Autodesk Inventor part; units mm, degrees
ref_plane "YZ Plane" through (0, 0, 0) normal (1, 0, 0) x (0, 1, 0)
ref_plane "XZ Plane" through (0, 0, 0) normal (0, 1, 0) x (-1, 0, 0)
ref_plane "XY Plane" through (0, 0, 0) normal (0, 0, 1) x (1, 0, 0)
sketch "Sketch1" plane through (0, 0, 0) normal (0, 1, 0) x (-1, 0, 0)
  circle A0 centre (0, 0) radius 3
  circle A1 centre (0, 0) radius 1.5
  circle A2 centre (0, 0) radius 1.75
  circle A3 centre (0, 0) radius 2.75
  dimension "d0" = 6
  dimension "d1" = 3
  dimension "d2" = 3.5
  dimension "d3" = 5.5
extrude "Extrusion1" add sketch "Sketch1" along normal blind 2.5 contours A0 | A2 | A3
extrude "Extrusion2" cut sketch "Sketch1" against normal blind 0.1 from surface at 2.5 contours A3
extrude "Extrusion3" cut sketch "Sketch1" along normal blind 0.1 contours A3
properties part number "Miniatur Kugellager MR 63 2RS 3x6x2.5 mm"
Verification items for the finished model (mm, model axes). A direction names the side the tool comes from. Give positions to 0.01 mm unless a question says otherwise; leave off trailing zeros. Order: outer loops, then holes, each group sorted by start corner. A loop starts at its lowest first (then second) coordinate and runs counter-clockwise, first axis right, second up. Notation, with made-up numbers: M 69.5,0 L 96.5,0 A5 cw 96.5,5 Z; hole C 57.25,82.5 d4. An arc over 180 degrees is marked long. Use one line per item in the form item = value. Start each with the question number.
Q1. Section check D-D (x = -1.95). Enter the section's corners in (y, z).
Q2. Go/stop test with a flat-tipped pin: pin 1 Ø1 at (y, z) = (0.5, 2) entering from +X. Record where the tip stops, or that it passes through.
Q3. Section check C-C (y = 1). Enter the section's corners in (x, z), then the cut area to 3 significant figures.
Q4. Section check B-B (x = 0). Enter the section's corners in (y, z), then the cut area to 3 significant figures.
Q5. Mould release check, pull along Z, two halves, no side actions. Record for faces 1 (the cylindrical face through (3, 1, 0)), 2 (the flat face through (-2, 0.1, 0)): +Z half, -Z half, draft (parallel to the pull), parting line (faces both ways), or undercut.
Q6. Access from +Z, -Z, +X, -X, +Y, -Y to the whole of each face (thin tool, end or side, straight path). Record for faces 3 (the flat face through (-2, 2.4, 0)), 4 (the cylindrical face through (1.5, 1.23, -0.07)).
Q7. Scan lines: line 1 along Z through (x, y) = (0, 0.05); line 2 along Z through (x, y) = (0, 0.15). Record each from-to range of solid material in increasing order. Write a range as [from, to].
Q8. Section check A-A (z = 0). Enter the section's corners in (x, y).
Evaluation:
q1.outline = M 0,-2.28 L 2.5,-2.28 L 2.5,-1.94 L 2.4,-1.94 L 2.4,1.94 L 2.5,1.94 L 2.5,2.28 L 0,2.28 L 0,1.94 L 0.1,1.94 L 0.1,-1.94 L 0,-1.94 Z
q2.pin_1 = 2.6
q3.outline = C 0,0 d6; hole C 0,0 d3
q3.area = 21.2 mm2
q4.outline = M 0,-3 L 2.5,-3 L 2.5,-2.75 L 2.4,-2.75 L 2.4,-1.75 L 2.5,-1.75 L 2.5,-1.5 L 0,-1.5 L 0,-1.75 L 0.1,-1.75 L 0.1,-2.75 L 0,-2.75 Z; M 0,1.5 L 2.5,1.5 L 2.5,1.75 L 2.4,1.75 L 2.4,2.75 L 2.5,2.75 L 2.5,3 L 0,3 L 0,2.75 L 0.1,2.75 L 0.1,1.75 L 0,1.75 Z
q4.area = 7.10 mm2
q5.face_1 = parting line
q5.face_2 = undercut
q6.face_3 = +Y
q6.face_4 = +Y, -Y
q7.line_1 = [-3, -2.75], [-1.75, -1.5], [1.5, 1.75], [2.75, 3]
q7.line_2 = [-3, -1.5], [1.5, 3]
q8.outline = M -3,0 L -2.75,0 L -2.75,0.1 L -1.75,0.1 L -1.75,0 L -1.5,0 L -1.5,2.5 L -1.75,2.5 L -1.75,2.4 L -2.75,2.4 L -2.75,2.5 L -3,2.5 Z; M 1.5,0 L 1.75,0 L 1.75,0.1 L 2.75,0.1 L 2.75,0 L 3,0 L 3,2.5 L 2.75,2.5 L 2.75,2.4 L 1.75,2.4 L 1.75,2.5 L 1.5,2.5 Z
